Verification items for the finished model (mm, model axes). Face numbers are marked on the shaded views. A direction names the side the tool comes from. Round coordinates to 2 decimals unless told otherwise and drop trailing zeros. Write each loop counter-clockwise with the first axis right and the second up, starting at its lowest first coordinate (ties: lowest second). Pieces come first, ordered by that corner, then holes. Notation, with made-up numbers: (23, -1.5) -> (60, -1.5) arc R22 ccw to (60, 24.5) -> close; hole circle Ø7 at (3, 83.25). An arc over 180 degrees is marked (long way). Use CSV: the item, a comma, the result in double quotes.
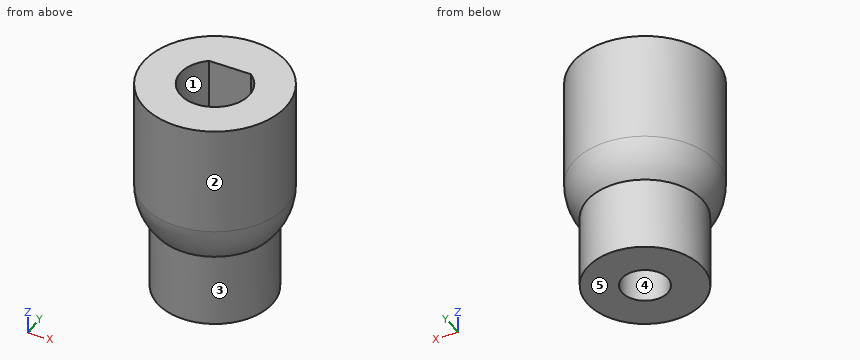
```python
from build123d import *

# Parameters (mm, degrees)
SKETCH1_R           = 6.1722
BOSS_EXTRUDE1_DEPTH = 12.7
SKETCH2_R           = 4.985
SKETCH2_R_2         = 1.985
BOSS_EXTRUDE2_DEPTH = 6.35
FILLET1_R           = 5


with BuildPart() as part:
    # Sketch1 → Boss-Extrude1 (new body)
    with BuildSketch(Plane.XY):
        Circle(SKETCH1_R)
        with BuildLine():
            Line((-1.8034, 2.393941578), (1.8034, 2.393941578))
            ThreePointArc((1.8034, 2.393941578), (0, -2.9972), (-1.8034, 2.393941578))
        make_face(mode=Mode.SUBTRACT)
    extrude(amount=BOSS_EXTRUDE1_DEPTH)

    # Sketch2 → Boss-Extrude2 (add)
    with BuildSketch(Plane(origin=(0, 0, 0), x_dir=(-1, 0, 0), z_dir=(0, 0, -1))):
        Circle(SKETCH2_R)
        Circle(SKETCH2_R_2, mode=Mode.SUBTRACT)
    extrude(amount=BOSS_EXTRUDE2_DEPTH)

    # Fillet1
    # the kernel refuses this fillet: 5 mm, written as the material it takes off along each edge
    with BuildSketch(Plane(origin=(0, 0, 0), x_dir=(1, 0, 0), z_dir=(0, -1, 0))) as fillet1_piece_1_section:
        with BuildLine():
            CenterArc((1.1722, 3.234587479), FILLET1_R, 319.690404577, 40.309595423)
            Line((4.985, 0), (5.061256, -0.06469175))
            ThreePointArc((5.061256, -0.06469175), (5.5786, -0.1), (6.1722, -0.1))
            Line((6.1722, -0.1), (6.2722, 0))
            Line((6.2722, 0), (6.2722, 3.234587479))
            Line((6.2722, 3.234587479), (6.1722, 3.234587479))
        make_face()
    fillet1_piece_1 = revolve(axis=Axis((0, 0, 0), (0, 0, 1)), mode=Mode.PRIVATE)
    fillet1_piece_1 = fillet1_piece_1 - Plane(origin=(0, 0, 1.498233037), x_dir=(-1, 0, 0), z_dir=(0, 0, 1)) * Cylinder(4.985, 26, mode=Mode.PRIVATE)
    add(fillet1_piece_1, mode=Mode.SUBTRACT)


solid = part.part
```
Q1. Section check B-B (z = 4.25). Record the cut outline in (x, y).
Filled in:
outline,"circle Ø12.34 at (0, 0); hole (-1.8, 2.39) arc R3 ccw (long way) to (1.8, 2.39) -> close"
Q2. Access from +Z, -Z, +X, -X, +Y, -Y to the whole of each face (thin tool, end or side, straight path). Record for the marked faces 1 and 2.
Filled in:
face 1,"+Z"
face 2,"+Z, -Z"
Q3. Material ranges on L1, parallel to Y at x = 0, z = 3.5; L2, parallel to Y at x = 0, z = -3 (3 decimals); L3, parallel to X at y = -1.5, z = 0.25, recorded low to high.
Filled in:
L1,"-6.17 to -3, 2.39 to 6.17"
L2,"-4.985 to -1.985, 1.985 to 4.985"
L3,"-4.96 to -2.59, 2.59 to 4.96"
Q4. Section check A-A (z = -0.5). Record the cut outline in (x, y) (3 decimals), plus the area to 3 significant figures.
Filled in:
outline,"circle Ø9.97 at (0, 0); hole circle Ø3.97 at (0, 0)"
area,"65.7 mm²"
Q5. Go/stop test with flat-tipped pins: P1, Ø6, axis at x = 5, z = -0.5, coming from the +Y side; P2, Ø3, axis at x = 4, z = 1, coming from the +Y side. Record where each tip stops, or that it passes through.
Filled in:
P1,"y = 5.17"
P2,"y = 5.3"
Q6. Mould release check, pull along Y, two halves, no side actions. Record for the marked faces 3, 4 and 5: released by +Y, released by -Y, zero draft, split by the parting line, or undercut.
Filled in:
face 3,"split by the parting line"
face 4,"undercut"
face 5,"zero draft"
